Drawing for the job (mm, zero at the part's lowest x, y, z). A direction names the side the tool comes from. Round coordinates to 2 decimals unless told otherwise and drop trailing zeros. Loops run counter-clockwise (first coordinate to the right, second up) from the corner with the lowest first, then second, coordinate; pieces in that order, holes last. Notation, with made-up numbers: M 58,-9.75 L 89,-9.75 A28 cw 89,14.25 Z; hole C 38.5,22.25 d3. An arc over 180 degrees is marked long. Use a Markdown table: item, result. Add a question column.
Q1. Cut at C-C (x = 40). Give the cut face in (y, z).
Q2. Cut at B-B (y = 3.25). Give the cut face in (x, z).
Q3. Tool access for the marked faces 1 and 2: list every direction of +Z, -Z, +X, -X, +Y, -Y with a clear straight run to the whole face (end or side of a thin tool).
Q4. Cut at D-D (y = 15). Give the cut face in (x, z), plus the area to 3 significant figures.
Q5. Probe line 1 (X direction, y = 8.5, z = 25); line 2 (Z direction, x = 40, y = 7.5); line 3 (Y direction, x = 7, z = 19). List the from-to ranges inside material, lowest first. Write a range as from..to.
Q6. Pin check, flat tips, straight feed: pin 1 (8 mm diameter, centred on x = 10, z = 25, fed in from -Y); pin 2 (14.5 mm diameter, centred on x = 70, z = 25, fed in from +Y); pin 3 (1 mm diameter, centred on y = 6, z = 7, fed in from +X); pin 4 (5 mm diameter, centred on x = 10.5, y = 5, fed in from +Z). Stop position of each tip, or through.
Q7. Cut at A-A (x = 8.5). Give the cut face in (y, z).
Q8. Mould opens along X. For the marked faces 3, 4 and 5 say: +X half, -X half, draft (parallel to the pull), parting line (faces both ways), or undercut.
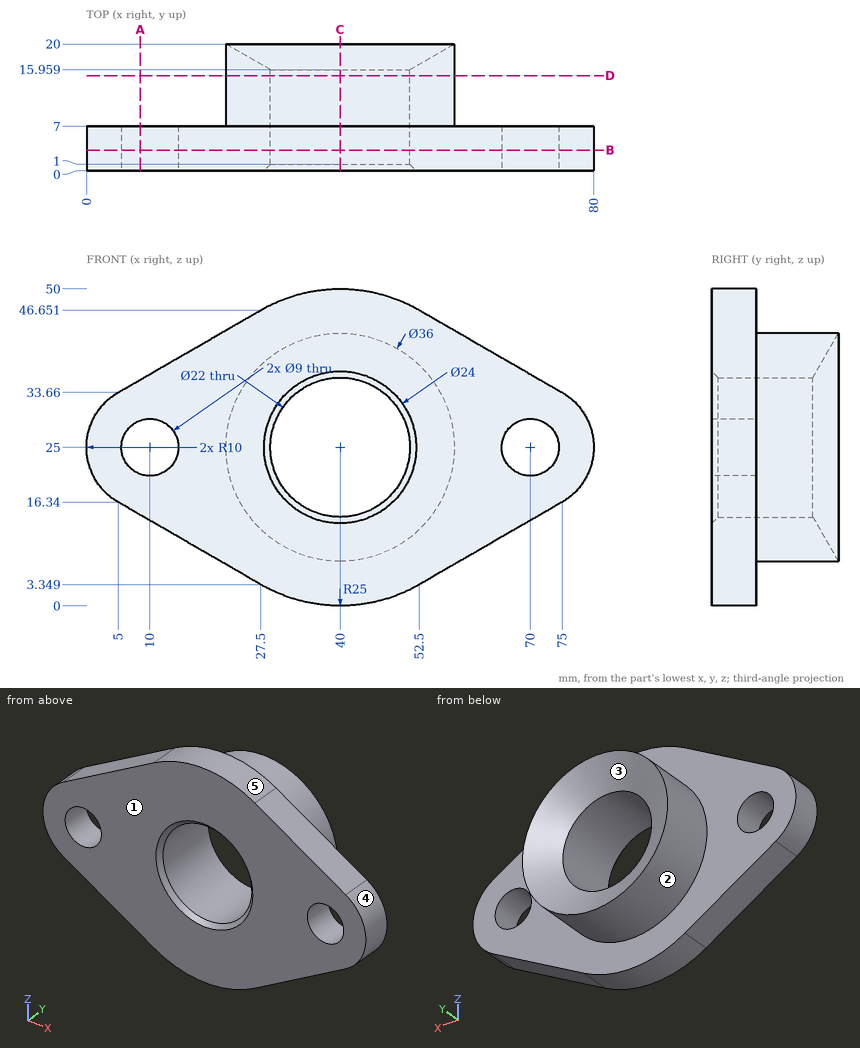
Checked values:
| question | item | result |
|---|---|---|
| 1 | outline | M 0,0 L 7,0 L 7,7 L 20,7 L 15.96,14 L 1,14 L 0,13 Z; M 0,37 L 1,36 L 15.96,36 L 20,43 L 7,43 L 7,50 L 0,50 Z |
| 2 | outline | M 5,16.34 L 27.5,3.35 A25 ccw 52.5,3.35 L 75,16.34 A10 ccw 75,33.66 L 52.5,46.65 A25 ccw 27.5,46.65 L 5,33.66 A10 ccw Z; hole C 10,25 d9; hole C 40,25 d22; hole C 70,25 d9 |
| 3 | face 1 | +Z, -Z, +X, -X, -Y |
| 3 | face 2 | +Y |
| 4 | outline | C 40,25 d36; hole C 40,25 d22 |
| 4 | area | 638 mm^2 |
| 5 | line 1 | x = 22..29, 51..58 |
| 5 | line 2 | z = 7..14, 36..43 |
| 5 | line 3 | y = 0..7 |
| 6 | pin 1 | passes through |
| 6 | pin 2 | stops at y = 7 |
| 6 | pin 3 | stops at x = 59.69 |
| 6 | pin 4 | stops at z = 38.28 |
| 7 | outline | M 0,14.32 L 7,14.32 L 7,20.76 L 0,20.76 Z; M 0,29.24 L 7,29.24 L 7,35.68 L 0,35.68 Z |
| 8 | face 3 | undercut |
| 8 | face 4 | +X half |
| 8 | face 5 | parting line |
